Source: CAD feature listing. Evaluate the final solid. Frame: model axes, mm. Round coordinates to 2 decimals unless told otherwise and drop trailing zeros. Order: outer loops, then holes, each group sorted by start corner. A loop starts at its lowest first (then second) coordinate and runs counter-clockwise, first axis right, second up. Notation, with made-up numbers: (-20, -33.5) - (24, -33.5) arc R22 ccw to (24, -26.5) - close; hole circle Ø11 at (9.5, 46). An arc over 180 degrees is marked (long way). Use one line per item in the form item = value. Start each with the question number.
Q1. Cut plane B-B, the plane x = -15. Return the cut outline in (y, z).
Q2. Pin query (flat end, axial travel): pin 1 Ø1 at (x, y) = (-9, -12) entering from -Z; pin 2 Ø5.5 at (x, y) = (25.4, -25.4) entering from +Z. Return the tip coordinate at first contact, or that it passes through.
Q3. Cut plane C-C, the plane z = 2. Give the number of separate pieces and of enclosed holes in the cut face, and give its area (3 significant figures).
Q4. Ray query, line 1 (Y direction, x = -15, z = 5); line 2 (Y direction, x = -25.4, z = 1.75) (3 decimals); line 3 (X direction, y = 25, z = 3.5). Return the intervals inside material, ascending. Write a range as [from, to].
Q5. Draft query along X for faces 1 (the flat face through (0, -31, 3)), 2 (the flat face through (30, 0, 3)), 3 (the flat face through (-30, 0, 3)), 4 (the cylindrical face through (28.43, 26.35, 3.13)). Return one class per face: released by +X, released by -X, zero draft, split by the parting line, or undercut.
Q6. Cut plane A-A, the plane y = -15. Return the cut outline in (x, z).
from build123d import *

# Parameters (mm, degrees)
SKETCH1_W           = 60
SKETCH1_H           = 62
SKETCH1_R           = 3.175
SKETCH1_R_2         = 2.071
BOSS_EXTRUDE1_DEPTH = 6.35


with BuildPart() as part:
    # Sketch1 → Boss-Extrude1 (new body)
    with BuildSketch(Plane.XY):
        Rectangle(SKETCH1_W, SKETCH1_H)
        with Locations((25.4, 25.4)):
            Circle(SKETCH1_R, mode=Mode.SUBTRACT)
        with Locations((-25.4, 25.4)):
            Circle(SKETCH1_R, mode=Mode.SUBTRACT)
        with Locations((25.4, -25.4)):
            Circle(SKETCH1_R, mode=Mode.SUBTRACT)
        with Locations((-25.4, -25.4)):
            Circle(SKETCH1_R, mode=Mode.SUBTRACT)
        with Locations((-15, 15)):
            Circle(SKETCH1_R_2, mode=Mode.SUBTRACT)
        with Locations((-15, -15)):
            Circle(SKETCH1_R_2, mode=Mode.SUBTRACT)
        with Locations((15, -15)):
            Circle(SKETCH1_R_2, mode=Mode.SUBTRACT)
        with Locations((15, 15)):
            Circle(SKETCH1_R_2, mode=Mode.SUBTRACT)
    extrude(amount=BOSS_EXTRUDE1_DEPTH)


solid = part.part
Completed:
q1.outline = (-31, 0) - (-17.07, 0) - (-17.07, 6.35) - (-31, 6.35) - close; (-12.93, 0) - (12.93, 0) - (12.93, 6.35) - (-12.93, 6.35) - close; (17.07, 0) - (31, 0) - (31, 6.35) - (17.07, 6.35) - close
q2.pin_1 = 0
q2.pin_2 = through
q3.separate_pieces = 1
q3.enclosed_holes = 8
q3.area = 3,540 mm2
q4.line_1 = [-31, -17.07], [-12.93, 12.93], [17.07, 31]
q4.line_2 = [-31, -28.575], [-22.225, 22.225], [28.575, 31]
q4.line_3 = [-30, -28.55], [-22.25, 22.25], [28.55, 30]
q5.face_1 = zero draft
q5.face_2 = released by +X
q5.face_3 = released by -X
q5.face_4 = undercut
q6.outline = (-30, 0) - (-17.07, 0) - (-17.07, 6.35) - (-30, 6.35) - close; (-12.93, 0) - (12.93, 0) - (12.93, 6.35) - (-12.93, 6.35) - close; (17.07, 0) - (30, 0) - (30, 6.35) - (17.07, 6.35) - close
